from build123d import *

# Parameters (mm, degrees)
SKETCH_1_R          = 21.5
SKETCH_1_R_2        = 2.15
SKETCH_1_R_3        = 9.7
EXTRUDE_1_DEPTH     = 5.5
SKETCH_2_R          = 10.9
SKETCH_2_R_2        = 9.55
CUT_EXTRUDE_1_DEPTH = 1.5
CUT_EXTRUDE_2_DEPTH = 31.899029111
SKETCH_4_R          = 4.5
CUT_EXTRUDE_3_DEPTH = 3.3


with BuildPart() as part:
    # 草图1 → 凸台-拉伸1 (new body)
    with BuildSketch(Plane.XY):
        Circle(SKETCH_1_R)
        with Locations((0, 17.5)):
            Circle(SKETCH_1_R_2, mode=Mode.SUBTRACT)
        with Locations((17.5, 0)):
            Circle(SKETCH_1_R_2, mode=Mode.SUBTRACT)
        with Locations((-17.5, 0)):
            Circle(SKETCH_1_R_2, mode=Mode.SUBTRACT)
        with Locations((0, -17.5)):
            Circle(SKETCH_1_R_2, mode=Mode.SUBTRACT)
        Circle(SKETCH_1_R_3, mode=Mode.SUBTRACT)
    extrude(amount=EXTRUDE_1_DEPTH)

    # 草图2 → 切除-拉伸1 (cut)
    with BuildSketch(Plane.XY.offset(5.5)):
        Circle(SKETCH_2_R)
        Circle(SKETCH_2_R_2, mode=Mode.SUBTRACT)
    extrude(amount=-CUT_EXTRUDE_1_DEPTH, mode=Mode.SUBTRACT)

    # 草图3 → 切除-拉伸2 (cut, through all)
    with BuildSketch(Plane.XY.offset(5.5)):
        with BuildLine():
            ThreePointArc((5.784529249, 20.707226308), (12.02081528, 12.02081528), (20.707226308, 5.784529249))
            ThreePointArc((20.707226308, 5.784529249), (15.202795796, 15.202795796), (5.784529249, 20.707226308))
        make_face()
        with BuildLine():
            ThreePointArc((-20.707226308, 5.784529249), (-12.02081528, 12.02081528), (-5.784529249, 20.707226308))
            ThreePointArc((-5.784529249, 20.707226308), (-15.202795796, 15.202795796), (-20.707226308, 5.784529249))
        make_face()
        with BuildLine():
            ThreePointArc((-5.784529249, -20.707226308), (-12.02081528, -12.02081528), (-20.707226308, -5.784529249))
            ThreePointArc((-20.707226308, -5.784529249), (-15.202795796, -15.202795796), (-5.784529249, -20.707226308))
        make_face()
        with BuildLine():
            ThreePointArc((20.707226308, -5.784529249), (12.02081528, -12.02081528), (5.784529249, -20.707226308))
            ThreePointArc((5.784529249, -20.707226308), (15.202795796, -15.202795796), (20.707226308, -5.784529249))
        make_face()
    extrude(amount=-CUT_EXTRUDE_2_DEPTH, mode=Mode.SUBTRACT)

    # 草图4 → 切除-拉伸3 (cut)
    with BuildSketch(Plane(origin=(0, 0, 0), x_dir=(-1, 0, 0), z_dir=(0, 0, -1))):
        with Locations((0, 17.5)):
            Circle(SKETCH_4_R)
        with Locations((17.5, 0)):
            Circle(SKETCH_4_R)
        with Locations((-17.5, 0)):
            Circle(SKETCH_4_R)
        with Locations((0, -17.5)):
            Circle(SKETCH_4_R)
    extrude(amount=-CUT_EXTRUDE_3_DEPTH, mode=Mode.SUBTRACT)


solid = part.part
Geometry check sheet. Reference: the model listing, model coordinates, mm. A direction names the side the tool comes from. Round coordinates to 2 decimals unless told otherwise and drop trailing zeros. Order: outer loops, then holes, each group sorted by start corner. A loop starts at its lowest first (then second) coordinate and runs counter-clockwise, first axis right, second up. Notation, with made-up numbers: M -34,7 L -13,7 A16 ccw -13,11 Z; hole C 42.25,85 d5. An arc over 180 degrees is marked long. Answer in a Markdown table with one row per item. Add a question column.
Item 1: Sectioned sample at A-A, the plane x = 0. Enter the section's corners in (y, z), plus the area to 3 significant figures.
Item 2: Sectioned sample at B-B, the plane y = -8.5. Enter the section's corners in (x, z).
Item 3: Sectioned sample at C-C, the plane z = 4.9. Enter the section's corners in (x, y).
Item 4: Draft check along Y on faces 1 (the face through (0, 13, 2)), 2 (the face through (12.13, -11.91, 2.79)), 3 (the face through (0.1, 21.5, 3.9)). Enter one of: released by +Y, released by -Y, zero draft, split by the parting line, or undercut.
Item 5: Sectioned sample at D-D, the plane x = -17.5. Enter the section's corners in (y, z), plus the area to 3 significant figures.
Item 6: Set-up check for faces 4 (the face through (10.4, 3.27, 4.76)), 5 (the face through (-11.91, -12.13, 2.79)), 6 (the face through (0, -15, 3.3)): record each of +Z, -Z, +X, -X, +Y, -Y from which the full face is reachable in a straight line by a thin tool's end or side.
Item 7: Material ranges on L1, parallel to Y at x = 0, z = 5.05; L2, parallel to X at y = 0, z = 3.55; L3, parallel to Y at x = 0, z = 0.7, recorded low to high. Write a range as [from, to].
Item 8: Depth check by flat-ended pin: pin 1 Ø1 at (x, y) = (-7, 15) entering from -Z; pin 2 Ø8 at (x, y) = (17.5, 0) entering from -Z. Enter the tip coordinate at first touch or a pass-through.
Filled in:
| question | item | result |
|---|---|---|
| 1 | outline | M -21.5,3.3 L -19.65,3.3 L -19.65,5.5 L -21.5,5.5 Z; M -15.35,3.3 L -13,3.3 L -13,0 L -9.7,0 L -9.7,4 L -10.9,4 L -10.9,5.5 L -15.35,5.5 Z; M 9.7,0 L 13,0 L 13,3.3 L 15.35,3.3 L 15.35,5.5 L 10.9,5.5 L 10.9,4 L 9.7,4 Z; M 19.65,3.3 L 21.5,3.3 L 21.5,5.5 L 19.65,5.5 Z |
| 1 | area | 51.2 mm² |
| 2 | outline | M -16.18,0 L -4.67,0 L -4.67,4 L -6.82,4 L -6.82,5.5 L -16.18,5.5 Z; M 4.67,0 L 16.18,0 L 16.18,5.5 L 6.82,5.5 L 6.82,4 L 4.67,4 Z |
| 3 | outline | M -20.71,-5.78 A33 cw -5.78,-20.71 A21.5 ccw 5.78,-20.71 A33 cw 20.71,-5.78 A21.5 ccw 20.71,5.78 A33 cw 5.78,20.71 A21.5 ccw -5.78,20.71 A33 cw -20.71,5.78 A21.5 ccw Z; hole C -17.5,0 d4.3; hole C 0,0 d21.8; hole C 0,-17.5 d4.3; hole C 0,17.5 d4.3; hole C 17.5,0 d4.3 |
| 4 | face 1 | undercut |
| 4 | face 2 | released by -Y |
| 4 | face 3 | released by +Y |
| 5 | outline | M -7.6,0 L -4.5,0 L -4.5,3.3 L -2.15,3.3 L -2.15,5.5 L -7.6,5.5 Z; M 2.15,3.3 L 4.5,3.3 L 4.5,0 L 7.6,0 L 7.6,5.5 L 2.15,5.5 Z |
| 5 | area | 44.5 mm² |
| 6 | face 4 | +Z |
| 6 | face 5 | +Z, -Z, -X, -Y |
| 6 | face 6 | -Z |
| 7 | L1 | y = [-21.5, -19.65], [-15.35, -10.9], [10.9, 15.35], [19.65, 21.5] |
| 7 | L2 | x = [-21.5, -19.65], [-15.35, -9.7], [9.7, 15.35], [19.65, 21.5] |
| 7 | L3 | y = [-13, -9.7], [9.7, 13] |
| 8 | pin 1 | stops at z = 0 |
| 8 | pin 2 | stops at z = 3.3 |
